For this review, take the finished solid that the model builds, in its own axes (mm). Coordinates: 2 decimals unless noted, no trailing zeros. Loops run counter-clockwise (first coordinate to the right, second up) from the corner with the lowest first, then second, coordinate; pieces in that order, holes last.
1. Take a section at C-C, the plane y = 1. State the section outline as (x, z) points, then the cut area to 3 significant figures.
2. To check wall thickness, follow probe 1 along Y at (x, z) = (-0.1, -32); probe 2 along Y at (x, z) = (-0.6, -30); probe 3 along X at (y, z) = (-1.4, -15.5). State the ranges of each line that lie inside material, in increasing order.
3. Take a section at A-A, the plane z = -3. State the section outline as (x, y) points.
4. Clearance check with flat-ended pins moving along their axes: P1, Ø2, axis at x = -1.5, y = 0.5, coming from the -Z side; P2, Ø1.5, axis at x = -1, z = -24, coming from the +Y side; P3, Ø2, axis at x = 1, y = 1.5, coming from the +Z side. State where each tip first meets the part, or that it passes through.
5. Take a section at B-B, the plane x = -1.25. State the section outline as (y, z) points.
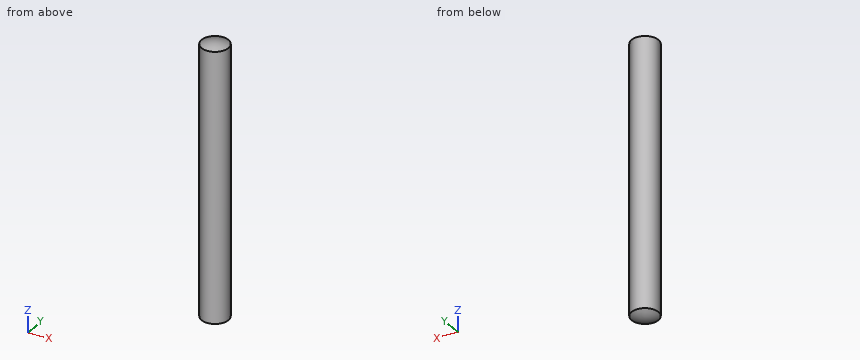
Autodesk Inventor part; units mm, degrees
ref_plane "YZ Plane" through (0, 0, 0) normal (1, 0, 0) x (0, 1, 0)
ref_plane "XZ Plane" through (0, 0, 0) normal (0, 1, 0) x (-1, 0, 0)
ref_plane "XY Plane" through (0, 0, 0) normal (0, 0, 1) x (1, 0, 0)
sketch "Sketch1" plane through (0, 0, 0) normal (0, 0, 1) x (1, 0, 0)
  circle A0 centre (0, 0) radius 2
  dimension "d0" = 4
extrude "Extrusion1" add sketch "Sketch1" against normal blind 40
sketch "Sketch3" plane through (0, 0, 0) normal (1, 0, 0) x (0, 1, 0)
  line L0 (0, 0) -> (0, 0.5)
  line L1 (2, 0) -> (-2, 0)
  arc A0 (2, 0) -> (0, 0.5) centre (0, -3.75) ccw
  line L2 (2, 0) -> (0, 0)
  dimension "d5" = 0.5
  dimension "d7" = 4.25
revolve "Revolution1" add sketch "Sketch3" angle 360 about axis through (0, 0, 0) along (0, 0, 1)
sketch "Sketch4" plane through (0, 0, 0) normal (1, 0, 0) x (0, 1, 0)
  line L0 (-2, -40) -> (2, -40)
  line L1 (0, -40) -> (0, -40.5)
  arc A0 (0, -40.5) -> (2, -40) centre (0, -36.25) ccw
  line L2 (2, -40) -> (0, -40)
  point P0 (0, 0)
  dimension "d9" = 0.5
  dimension "d11" = 4.25
revolve "Revolution2" add sketch "Sketch4" angle 360 about axis through (0, 0, -40) along (0, 0, -1)
properties part number "Poker hinge 3"
Results list:
1. outline: (-1.73, -40) arc R4.13 ccw to (1.73, -40) - (1.73, 0) arc R4.13 ccw to (-1.73, 0) - close
1. area: 140 mm2
2. probe 1: y = -2 to 2
2. probe 2: y = -1.91 to 1.91
2. probe 3: x = -1.43 to 1.43
3. outline: circle Ø4 at (0, 0)
4. P1: stops at z = -40.46
4. P2: stops at y = 1.98
4. P3: stops at z = 0.42
5. outline: (-1.56, -40) arc R4.06 ccw to (1.56, -40) - (1.56, 0) arc R4.06 ccw to (-1.56, 0) - close
